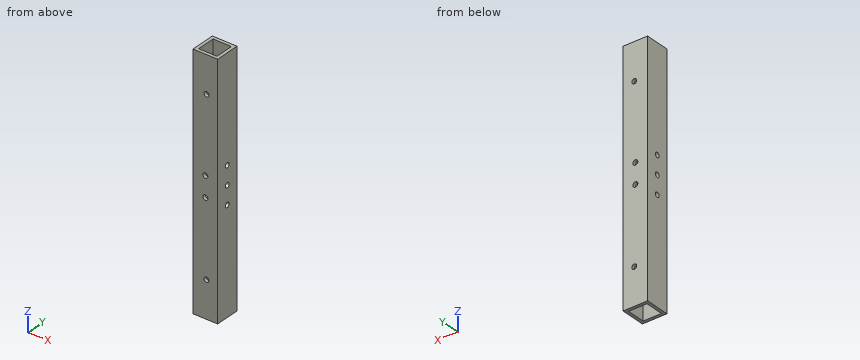
Autodesk Inventor part; units mm, degrees
ref_plane "YZ Plane" through (0, 0, 0) normal (1, 0, 0) x (0, 1, 0)
ref_plane "XZ Plane" through (0, 0, 0) normal (0, 1, 0) x (-1, 0, 0)
ref_plane "XY Plane" through (0, 0, 0) normal (0, 0, 1) x (1, 0, 0)
sketch "Sketch1" plane through (0, 0, 0) normal (0, 0, 1) x (1, 0, 0)
  line L0 (0, 0) -> (25.4, 0)
  line L1 (25.4, 0) -> (25.4, 25.4)
  line L2 (25.4, 25.4) -> (0, 25.4)
  line L3 (0, 25.4) -> (0, 0)
  line L4 (3.175, 22.225) -> (22.225, 22.225)
  line L5 (22.225, 22.225) -> (22.225, 3.175)
  line L6 (22.225, 3.175) -> (3.175, 3.175)
  line L7 (3.175, 3.175) -> (3.175, 22.225)
  dimension "d0" = 25.4
  dimension "d1" = 25.4
  dimension "d2" = 3.175
extrude "Extrusion1" add sketch "Sketch1" along normal blind 190.5 and the other way blind 12.7
sketch "Sketch2" plane through (0, 25.4, -12.7) normal (0, 1, 0) x (1, 0, 0)
  line L0 (13.8579, 0) -> (13.8579, -12.7) construction
  line L1 (13.8579, -203.2028) -> (13.8579, -190.5028) construction
  circle A0 centre (13.8579, -190.5028) radius 2.5797
  circle A1 centre (13.8579, -12.7) radius 2.5797
  point P0 (0, -12.7)
  dimension "d6" = 12.7
  dimension "d7" = 12.7
  dimension "d8" = 5.1594
  dimension "d9" = 5.1594
extrude "Extrusion2" cut sketch "Sketch2" against normal blind 152.4
sketch "Sketch3" plane through (0, 0, 190.5) normal (0, 0, 1) x (1, 0, 0)
  line L0 (3.175, 3.175) -> (3.175, 22.225)
  line L1 (22.225, 22.225) -> (22.225, 3.175)
  line L2 (22.225, 3.175) -> (3.175, 3.175)
  line L3 (3.175, 3.175) -> (3.175, 22.225)
  line L4 (3.175, 22.225) -> (22.225, 22.225)
  line L5 (0, 0) -> (25.4, 0)
  line L6 (25.4, 0) -> (25.4, 25.4)
  line L7 (25.4, 25.4) -> (0, 25.4)
  line L8 (0, 25.4) -> (0, 0)
extrude "Extrusion3" add sketch "Sketch3" along normal blind 25.4
sketch "Sketch4" plane through (0, 0, -12.7) normal (0, 0, -1) x (-1, 0, 0)
  line L0 (-22.225, 3.175) -> (-22.225, 22.225)
  line L1 (-22.225, 22.225) -> (-3.175, 22.225)
  line L2 (-3.175, 22.225) -> (-3.175, 3.175)
  line L3 (-3.175, 3.175) -> (-22.225, 3.175)
  line L4 (-25.4, 0) -> (0, 0)
  line L5 (0, 0) -> (0, 25.4)
  line L6 (0, 25.4) -> (-25.4, 25.4)
  line L7 (-25.4, 25.4) -> (-25.4, 0)
extrude "Extrusion4" add sketch "Sketch4" along normal blind 25.4
sketch "Sketch5" plane through (0, 25.4, 215.9) normal (0, 1, 0) x (1, 0, 0)
  line L0 (3.175, 0) -> (22.225, 0) construction
  line L1 (12.7, 0) -> (12.7, 116.459) construction
  line L2 (22.225, 254) -> (3.175, 254) construction
  line L3 (12.7, 254) -> (12.7, 137.541) construction
  circle A0 centre (12.7, 137.541) radius 2.5797
  circle A1 centre (12.7, 116.459) radius 2.5797
  point P0 (0, 215.9)
  dimension "d18" = 116.459
  dimension "d19" = 116.459
  dimension "d20" = 5.1594
  dimension "d21" = 5.1594
extrude "Extrusion5" cut sketch "Sketch5" against normal blind 50.8
sketch "Sketch6" plane through (25.4, 0, 215.9) normal (1, 0, 0) x (0, 0, -1)
  line L0 (254, 25.4) -> (0, 25.4) construction
  line L1 (127, 25.4) -> (127, 12.7) construction
  line L2 (127, 12.7) -> (146.05, 12.7) construction
  line L3 (127, 12.7) -> (107.95, 12.7) construction
  circle A0 centre (127, 12.7) radius 2.5797
  circle A1 centre (146.05, 12.7) radius 2.5797
  circle A2 centre (107.95, 12.7) radius 2.5797
  point P0 (215.9, 0)
  dimension "d24" = 12.7
  dimension "d25" = 19.05
  dimension "d26" = 19.05
  dimension "d27" = 5.1594
  dimension "d28" = 5.1594
  dimension "d29" = 5.1594
extrude "Extrusion6" cut sketch "Sketch6" against normal blind 25.4
properties part number "base mount"
Design review of the part built by this model. Coordinates are the model's own, in mm. Give positions to 0.01 mm unless a question says otherwise; leave off trailing zeros. Order: outer loops, then holes, each group sorted by start corner. A loop starts at its lowest first (then second) coordinate and runs counter-clockwise, first axis right, second up.
1. To check wall thickness, follow L1, parallel to X at y = 19.5, z = -2 (3 decimals); L2, parallel to Y at x = 23.2, z = 88.9. State the ranges of each line that lie inside material, in increasing order.
Solution:
L1: x = 0 to 3.175, 22.225 to 25.4
L2: y = 0 to 10.12, 15.28 to 25.4
2. Add section A-A, the plane z = 88.9. State the section outline as (x, y) points (3 decimals), then the cut area to 3 significant figures.
Solution:
outline: (0, 0) - (25.4, 0) - (25.4, 10.12) - (22.225, 10.12) - (22.225, 3.175) - (3.175, 3.175) - (3.175, 10.12) - (0, 10.12) - close; (0, 15.28) - (3.175, 15.28) - (3.175, 22.225) - (22.225, 22.225) - (22.225, 15.28) - (25.4, 15.28) - (25.4, 25.4) - (0, 25.4) - close
area: 249 mm2
3. Add section C-C, the plane z = 166. State the section outline as (x, y) points (3 decimals), then the cut area to 3 significant figures.
Solution:
outline: (0, 0) - (25.4, 0) - (25.4, 25.4) - (0, 25.4) - close; hole (3.175, 3.175) - (22.225, 3.175) - (22.225, 22.225) - (3.175, 22.225) - close
area: 282 mm2
4. Add section B-B, the plane y = 6.5. State the section outline as (x, z) points (3 decimals).
Solution:
outline: (0, -38.1) - (3.175, -38.1) - (3.175, 215.9) - (0, 215.9) - close; (22.225, -38.1) - (25.4, -38.1) - (25.4, 215.9) - (22.225, 215.9) - close
5. For pin 1 Ø4.5 at (y, z) = (12.7, 88.9) entering from +X, flat-tipped, find the tip position at first contact; note if it passes through.
Solution:
pin 1: passes through
